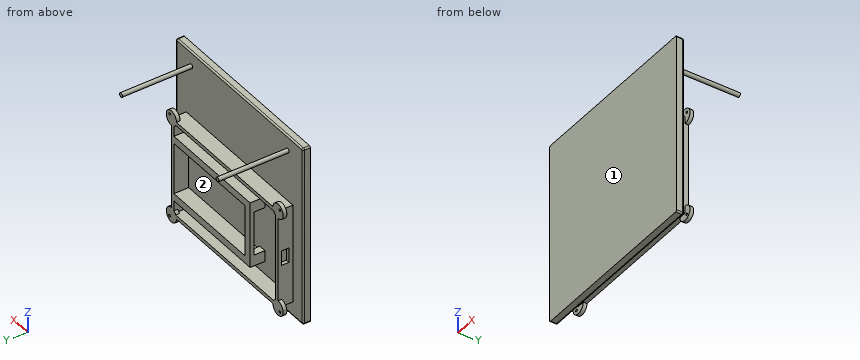
from build123d import *

# Parameters (mm, degrees)
SKETCH1_W           = 200
SKETCH1_H           = 125
BOSS_EXTRUDE3_DEPTH = 40
BOSS_EXTRUDE4_DEPTH = 10
EXTRUDE_THIN1_DEPTH = 40
SKETCH5_W           = 30
SKETCH5_H           = 15
CUT_EXTRUDE2_DEPTH  = 40
SKETCH6_W           = 210
SKETCH6_H           = 135
CUT_EXTRUDE3_DEPTH  = 20
SKETCH7_R           = 10
BOSS_EXTRUDE5_DEPTH = 5
SKETCH8_R           = 1.7
CUT_EXTRUDE5_DEPTH  = 5
SKETCH9_W           = 10
SKETCH9_H           = 5
CUT_EXTRUDE6_DEPTH  = 10
SKETCH10_W          = 230
SKETCH10_H          = 155
BOSS_EXTRUDE6_DEPTH = 10
SKETCH14_R          = 2.8
BOSS_EXTRUDE7_DEPTH = 95
FILLET1_R           = 2


with BuildPart() as part:
    # Sketch1 → Boss-Extrude3 (new body)
    with BuildSketch(Plane(origin=(0, 0, 0), x_dir=(1, 0, 0), z_dir=(0, 1, 0))):
        Polygon((5, 0), (0, 0), (0, -135), (210, -135), (210, 0), align=None)
        with Locations((105, -67.5)):
            Rectangle(SKETCH1_W, SKETCH1_H, mode=Mode.SUBTRACT)
    extrude(amount=BOSS_EXTRUDE3_DEPTH)

    # Sketch3 → Boss-Extrude4 (add)
    with BuildSketch(Plane(origin=(0, 0, 0), x_dir=(-1, 0, 0), z_dir=(0, -1, 0))):
        Polygon((-220, -145), (0, -145), (10, -145), (10, 10), (-220, 10), align=None)
    extrude(amount=BOSS_EXTRUDE4_DEPTH)

    # Sketch4 → Extrude-Thin1 (add)
    with BuildSketch(Plane(origin=(0, 0, 0), x_dir=(1, 0, 0), z_dir=(0, 1, 0))):
        Polygon((205, -32.5), (65, -32.5), (65, -102.5), (205, -102.5), (205, -112.5), (55, -112.5), (55, -22.5), (205, -22.5), align=None)
    extrude(amount=EXTRUDE_THIN1_DEPTH)

    # Sketch5 → Cut-Extrude2 (cut)
    with BuildSketch(Plane.ZY.offset(-55)):
        with Locations((82.5, 7.5)):
            Rectangle(SKETCH5_W, SKETCH5_H)
        with Locations((52.5, 7.5)):
            Rectangle(SKETCH5_W, SKETCH5_H)
    extrude(amount=-CUT_EXTRUDE2_DEPTH, mode=Mode.SUBTRACT)

    # Sketch6 → Cut-Extrude3 (cut)
    with BuildSketch(Plane(origin=(0, 40, 0), x_dir=(1, 0, 0), z_dir=(0, 1, 0))):
        with Locations((105, -67.5)):
            Rectangle(SKETCH6_W, SKETCH6_H)
    extrude(amount=-CUT_EXTRUDE3_DEPTH, mode=Mode.SUBTRACT)

    # Sketch7 → Boss-Extrude5 (add)
    with BuildSketch(Plane(origin=(0, 20, 0), x_dir=(1, 0, 0), z_dir=(0, 1, 0))):
        Circle(SKETCH7_R)
        with Locations((210, 0)):
            Circle(SKETCH7_R)
        with Locations((210, -135)):
            Circle(SKETCH7_R)
        with Locations((0, -135)):
            Circle(SKETCH7_R)
    extrude(amount=-BOSS_EXTRUDE5_DEPTH)

    # Sketch8 → Cut-Extrude5 (cut)
    with BuildSketch(Plane(origin=(0, 20, 0), x_dir=(1, 0, 0), z_dir=(0, 1, 0))):
        with Locations(Location((-3.535533906, 3.535533906, 0), (0, 0, 270))):
            Circle(SKETCH8_R)
        with Locations(Location((213.535533906, 3.535533906, 0), (0, 0, 270))):
            Circle(SKETCH8_R)
        with Locations(Location((213.535533906, -138.535533906, 0), (0, 0, 270))):
            Circle(SKETCH8_R)
        with Locations(Location((-3.535533906, -138.535533906, 0), (0, 0, 270))):
            Circle(SKETCH8_R)
    extrude(amount=-CUT_EXTRUDE5_DEPTH, mode=Mode.SUBTRACT)

    # Sketch9 → Cut-Extrude6 (cut)
    with BuildSketch(Plane.ZY):
        Polygon((77.5, 15.5), (77.5, 10.5), (67.5, 10.5), (57.5, 10.5), (57.5, 15.5), align=None)
        with Locations((72.5, 8)):
            Rectangle(SKETCH9_W, SKETCH9_H)
        with Locations((62.5, 8)):
            Rectangle(SKETCH9_W, SKETCH9_H)
    extrude(amount=-CUT_EXTRUDE6_DEPTH, mode=Mode.SUBTRACT)

    # Sketch10 → Boss-Extrude6 (add)
    with BuildSketch(Plane(origin=(0, 0, 0), x_dir=(1, 0, 0), z_dir=(0, 1, 0))):
        Polygon((230, 20), (-10, 20), (-20, 20), (-20, -225), (230, -225), align=None)
        with Locations((105, -67.5)):
            Rectangle(SKETCH10_W, SKETCH10_H, mode=Mode.SUBTRACT)
    extrude(amount=-BOSS_EXTRUDE6_DEPTH)

    # Sketch14 → Boss-Extrude7 (add)
    with BuildSketch(Plane(origin=(0, 0, 0), x_dir=(1, 0, 0), z_dir=(0, 1, 0))):
        with Locations(Location((10, -205, 0), (0, 0, 90))):
            Circle(SKETCH14_R)
        with Locations(Location((200, -205, 0), (0, 0, 90))):
            Circle(SKETCH14_R)
    extrude(amount=BOSS_EXTRUDE7_DEPTH)

    # Fillet1
    fillet1_edges = [part.edges().sort_by_distance(p)[0] for p in [
        (230, 0, 102.5),
        (230, -5, -20),
        (105, 0, 225),
        (230, -5, 225),
        (-20, 0, 102.5),
        (-20, -5, 225),
        (105, 0, -20),
        (-20, -5, -20),
    ]]
    fillet(fillet1_edges, radius=FILLET1_R)


solid = part.part
Here's how the part is built. I have some questions about the finished solid (model axes, mm). Face numbers are marked on the shaded views. Give positions to 0.01 mm unless a question says otherwise; leave off trailing zeros. Order: outer loops, then holes, each group sorted by start corner. A loop starts at its lowest first (then second) coordinate and runs counter-clockwise, first axis right, second up. Notation, with made-up numbers: (85, -7.75) -> (107, -7.75) arc R26 ccw to (107, 20.25) -> close; hole circle Ø10 at (71, 27.25). An arc over 180 degrees is marked (long way). Use a Markdown table: item, result. Add a question column.
Item 1: Will these pins go through, and if not, where does the flat tip stop? pin 1 (6 mm diameter, centred on x = 114, y = 5.5, fed in from +Z); pin 2 (6 mm diameter, centred on y = 10, z = 69, fed in from +X); pin 3 (6 mm diameter, centred on y = 5.5, z = 61.5, fed in from -X).
Item 2: Imagine slicing it at A-A on z = 45.5. Please give me the cut outline in (x, y), plus the area to 3 significant figures.
Item 3: I need wall thicknesses on line 1 (Z direction, x = 135, y = 14.5); line 2 (Y direction, x = 126, z = 137); line 3 (Z direction, x = 50, y = 2.5). Which ranges of each line are inside material? Lowest first, please.
Item 4: Imagine slicing it at C-C on x = 50. Please give me the cut outline in (y, z), plus the area to 3 significant figures.
Item 5: Imagine slicing it at D-D on y = 30.5. Please give me the cut outline in (x, z).
Item 6: If we mould it in two halves opening along Z, with no side actions, what happens to the marked faces 1 and 2? For each: pulls with the +Z half, pulls with the -Z half, needs draft (parallel to the pull), parting line crosses it, or undercut.
Item 7: Imagine slicing it at B-B on z = 169.5. Please give me the cut outline in (x, y).
Data:
| question | item | result |
|---|---|---|
| 1 | pin 1 | stops at z = 135 |
| 1 | pin 2 | stops at x = 210 |
| 1 | pin 3 | stops at x = 0 |
| 2 | outline | (-20, -10) -> (230, -10) -> (230, -2) arc R2 ccw to (228, 0) -> (210, 0) -> (210, 20) -> (205, 20) -> (205, 0) -> (5, 0) -> (5, 20) -> (0, 20) -> (0, 0) -> (-18, 0) arc R2 ccw to (-20, -2) -> close; (55, 15) -> (65, 15) -> (65, 20) -> (55, 20) -> close |
| 2 | area | 2,750 mm² |
| 3 | line 1 | z = 0 to 5, 22.5 to 32.5, 102.5 to 112.5, 130 to 135 |
| 3 | line 2 | y = -10 to 0 |
| 3 | line 3 | z = 0 to 5, 130 to 135 |
| 4 | outline | (-10, -20) -> (-2, -20) arc R2 ccw to (0, -18) -> (0, 0) -> (20, 0) -> (20, 5) -> (0, 5) -> (0, 130) -> (20, 130) -> (20, 135) -> (0, 135) -> (0, 223) arc R2 ccw to (-2, 225) -> (-10, 225) -> close |
| 4 | area | 2,650 mm² |
| 5 | outline | circle Ø5.6 at (10, 205); circle Ø5.6 at (200, 205) |
| 6 | face 1 | needs draft |
| 6 | face 2 | undercut |
| 7 | outline | (-20, -10) -> (230, -10) -> (230, -2) arc R2 ccw to (228, 0) -> (-18, 0) arc R2 ccw to (-20, -2) -> close |
